Source: CAD feature listing. Evaluate the final solid. Frame: model axes, mm. Face numbers are marked on the shaded views. Give positions to 0.01 mm unless a question says otherwise; leave off trailing zeros. Loops run counter-clockwise (first coordinate to the right, second up) from the corner with the lowest first, then second, coordinate; pieces in that order, holes last. Notation, with made-up numbers: M 3,58 L 52,58 A33 cw 52,97 Z; hole C 60.5,4 d2. An arc over 180 degrees is marked long. Put each result on its own line as item: value.
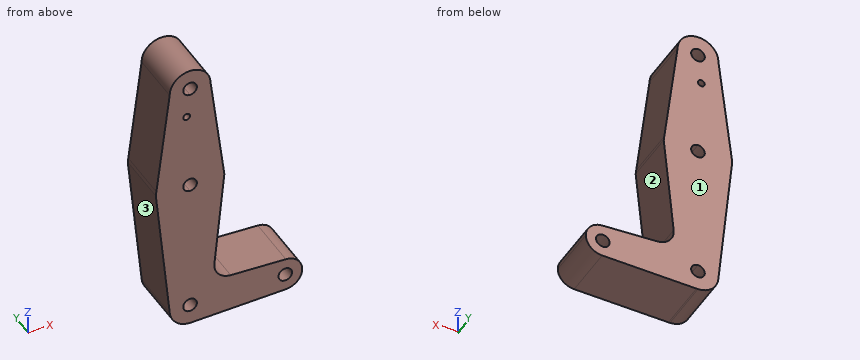
from build123d import *

# Parameters (mm, degrees)
F0_R     = 1.5875
F1_DEPTH = 25.4


with BuildPart() as f1:
    # F0 (on Front) → F1 (new body)
    with BuildSketch(Plane.XZ):
        with BuildLine():
            ThreePointArc((0, -3.175), (-3.175, 0), (0, 3.175))
            Line((0, 3.175), (0, 15.875))
            ThreePointArc((0, 15.875), (-10.4901713759, 11.9151974178), (-15.7470819389, 2.0112273392))
            ThreePointArc((-15.7470819389, 2.0112273392), (-11.9151974178, -10.4901713759), (0, -15.875))
            Line((0, -15.875), (0, -3.175))
        make_face()
        with BuildLine():
            Line((0, 15.875), (0, 3.175))
            ThreePointArc((0, 3.175), (2.2450640303, 2.2450640303), (3.175, 0))
            ThreePointArc((3.175, 0), (2.2450640303, -2.2450640303), (0, -3.175))
            Line((0, -3.175), (0, -15.875))
            ThreePointArc((0, -15.875), (11.2253201513, -11.2253201513), (15.875, 0))
            ThreePointArc((15.875, 0), (15.8433599301, 1.0017839713), (15.7485658425, 1.9995746809))
            ThreePointArc((15.7485658425, 1.9995746809), (10.4945790039, 11.9113154828), (0, 15.875))
        make_face()
        with BuildLine():
            ThreePointArc((-15.7470819389, 2.0112273392), (-10.4901713759, 11.9151974178), (0, 15.875))
            Line((0, 15.875), (0, 36.5252))
            Line((0, 36.5252), (0, 41.275))
            ThreePointArc((0, 41.275), (-6.7102581313, 44.0399659164), (-9.5247398797, 50.7296066537))
            Line((-9.5247398797, 50.7296066537), (-15.7470819389, 2.0112273392))
        make_face()
        with Locations((-1.5875, 36.5252)):
            Circle(F0_R, mode=Mode.SUBTRACT)
        with BuildLine():
            Line((0, 36.5252), (0, 15.875))
            ThreePointArc((0, 15.875), (10.4945790039, 11.9113154828), (15.7485658425, 1.9995746809))
            Line((15.7485658425, 1.9995746809), (9.5219777707, 51.0399256846))
            ThreePointArc((9.5219777707, 51.0399256846), (9.5242444127, 50.9199723593), (9.525, 50.8))
            ThreePointArc((9.525, 50.8), (6.7351920908, 44.0648079092), (0, 41.275))
            Line((0, 41.275), (0, 36.5252))
        make_face()
        with BuildLine():
            ThreePointArc((15.875, 0), (11.2253201513, -11.2253201513), (0, -15.875))
            Line((0, -15.875), (0, -53.975))
            ThreePointArc((0, -53.975), (6.7351920908, -56.7648079092), (9.525, -63.5))
            Line((9.525, -63.5), (36.5125, -63.5))
            ThreePointArc((36.5125, -63.5), (38.9380895153, -57.7883672161), (44.7324052746, -55.5675253854))
            Line((44.7324052746, -55.5675253854), (18.9819405343, -54.6507790461))
            ThreePointArc((18.9819405343, -54.6507790461), (13.2729113611, -51.9308376972), (11.3550302967, -45.9048251463))
            Line((11.3550302967, -45.9048251463), (16.0024491774, 0))
            Line((16.0024491774, 0), (15.7485658425, 1.9995746809))
            ThreePointArc((15.7485658425, 1.9995746809), (15.8433599301, 1.0017839713), (15.875, 0))
        make_face()
        with BuildLine():
            Line((0, -53.975), (0, -15.875))
            ThreePointArc((0, -15.875), (-11.9151974178, -10.4901713759), (-15.7470819389, 2.0112273392))
            Line((-15.7470819389, 2.0112273392), (-16.0039571601, 0))
            Line((-16.0039571601, 0), (-9.4765361199, -64.4596291825))
            ThreePointArc((-9.4765361199, -64.4596291825), (-7.0663318972, -57.1130931964), (0, -53.975))
        make_face()
        with BuildLine():
            Line((0, -60.325), (0, -53.975))
            ThreePointArc((0, -53.975), (-7.0663318972, -57.1130931964), (-9.4765361199, -64.4596291825))
            ThreePointArc((-9.4765361199, -64.4596291825), (-6.3869068036, -70.5663318972), (0, -73.025))
            Line((0, -73.025), (0.6773435479, -73.000885786))
            ThreePointArc((0.6773435479, -73.000885786), (6.9705567315, -69.9912990883), (9.525, -63.5))
            Line((9.525, -63.5), (3.175, -63.5))
            ThreePointArc((3.175, -63.5), (-2.2450640303, -65.7450640303), (0, -60.325))
        make_face()
        with BuildLine():
            ThreePointArc((-9.5247398797, 50.7296066537), (-6.7102581313, 44.0399659164), (0, 41.275))
            ThreePointArc((0, 41.275), (6.7351920908, 44.0648079092), (9.525, 50.8))
            ThreePointArc((9.525, 50.8), (9.5242444127, 50.9199723593), (9.5219777707, 51.0399256846))
            ThreePointArc((9.5219777707, 51.0399256846), (-0.1551656616, 60.323736064), (-9.5247398797, 50.7296066537))
        make_face()
        with BuildLine():
            ThreePointArc((3.175, 50.8), (2.2450640303, 48.5549359697), (0, 47.625))
            ThreePointArc((0, 47.625), (-2.2450640303, 53.0450640303), (3.175, 50.8))
        make_face(mode=Mode.SUBTRACT)
        with BuildLine():
            Line((36.5125, -63.5), (9.525, -63.5))
            ThreePointArc((9.525, -63.5), (6.9705567315, -69.9912990883), (0.6773435479, -73.000885786))
            Line((0.6773435479, -73.000885786), (44.7324052746, -71.4324746146))
            ThreePointArc((44.7324052746, -71.4324746146), (38.9380895153, -69.2116327839), (36.5125, -63.5))
        make_face()
        with BuildLine():
            ThreePointArc((44.7324052746, -55.5675253854), (38.9380895153, -57.7883672161), (36.5125, -63.5))
            ThreePointArc((36.5125, -63.5), (38.9380895153, -69.2116327839), (44.7324052746, -71.4324746146))
            ThreePointArc((44.7324052746, -71.4324746146), (50.1616327839, -69.0119104847), (52.3875, -63.5))
            ThreePointArc((52.3875, -63.5), (50.1616327839, -57.9880895153), (44.7324052746, -55.5675253854))
        make_face()
        with BuildLine():
            ThreePointArc((47.625, -63.5), (44.45, -66.675), (41.275, -63.5))
            ThreePointArc((41.275, -63.5), (44.45, -60.325), (47.625, -63.5))
        make_face(mode=Mode.SUBTRACT)
        with BuildLine():
            ThreePointArc((0, -73.025), (0.3388863295, -73.0189695375), (0.6773435479, -73.000885786))
            Line((0.6773435479, -73.000885786), (0, -73.025))
        make_face()
        with BuildLine():
            ThreePointArc((9.525, -63.5), (6.7351920908, -56.7648079092), (0, -53.975))
            Line((0, -53.975), (0, -60.325))
            ThreePointArc((0, -60.325), (2.2450640303, -61.2549359697), (3.175, -63.5))
            Line((3.175, -63.5), (9.525, -63.5))
        make_face()
    extrude(amount=F1_DEPTH)


solid = f1.part
1. Draft query along Z for the marked faces 1, 2 and 3. Return one class per face: pulls with the +Z half, pulls with the -Z half, needs draft (parallel to the pull), parting line crosses it, or undercut.
Found:
face 1: needs draft
face 2: undercut
face 3: pulls with the -Z half
2. Section query B-B (y = -20.5). State how many separate pieces and enclosed holes the cut face has, plus the area to 3 significant figures.
Found:
separate pieces: 1
enclosed holes: 5
area: 3,800 mm^2
3. Section query A-A (x = 43). Output: boundary loops of the cut face in (y, z), plus the area to 3 significant figures.
Found:
outline: M -25.4,-71.49 L 0,-71.49 L 0,-66.32 L -25.4,-66.32 Z; M -25.4,-60.68 L 0,-60.68 L 0,-55.51 L -25.4,-55.51 Z
area: 263 mm^2
4. Section query D-D (x = 29). Output: boundary loops of the cut face in (y, z).
Found:
outline: M -25.4,-71.99 L 0,-71.99 L 0,-55.01 L -25.4,-55.01 Z
5. Material intervals for line 1 (Z direction, x = 44.45, y = -6.75) (3 decimals); line 2 (X direction, y = -4.75, z = 50.8) (3 decimals); line 3 (X direction, y = -17, z = -63.5) (1 decimal), sorted ascending. Write a range as from..to.
Found:
line 1: -71.443..-66.675, -60.325..-55.557
line 2: -9.525..-3.175, 3.175..9.552
line 3: -9.6..-3.2, 3.2..41.3, 47.6..52.4
6. Contact query for flat-ended pins moving along their axis: P1, Ø1.5, axis at x = -3, y = -11.5, coming from the -Z side; P2, Ø8, axis at x = 44.5, y = -16.5, coming from the +Z side; P3, Ø8, axis at y = -7, z = 25, coming from the -X side. Output: stop coordinate, or through.
Found:
P1: z = -72.76
P2: z = -55.42
P3: x = -13.32
7. Section query C-C (z = 8). Output: boundary loops of the cut face in (x, y), plus the area to 3 significant figures.
Found:
outline: M -14.98,-25.4 L 14.99,-25.4 L 14.99,0 L -14.98,0 Z
area: 761 mm^2
